from build123d import *

# Parameters (mm, degrees)
SKETCH1_R           = 1.575
SKETCH1_W           = 3
SKETCH1_H           = 8
BOSS_EXTRUDE1_DEPTH = 3
SKETCH1_3_W         = 3
SKETCH1_3_H         = 8
SKETCH1_3_W_2       = 1.7
BOSS_EXTRUDE2_DEPTH = 15
SKETCH1_4_W         = 11.6
SKETCH1_4_H         = 3
BOSS_EXTRUDE3_DEPTH = 3.8
FILLET1_R           = 3


with BuildPart() as part:
    # Sketch1 → Boss-Extrude1 (new body)
    with BuildSketch(Plane(origin=(0, 0, 0), x_dir=(1, 0, 0), z_dir=(0, 1, 0))):
        Polygon((-13.5, -21.27), (-19.3, -28.36), (13.5, -28.36), (13.5, -20.375), (11.8, -20.375), (11.8, -12.375), (13.5, -12.375), (13.5, 12.375), (11.8, 12.375), (11.8, 20.375), (13.5, 20.375), (13.5, 28.36), (-19.3, 28.36), (-13.5, 21.27), align=None)
        with Locations(Location((-8.738402562, -18, 0), (0, 0, 270))):
            Circle(SKETCH1_R, mode=Mode.SUBTRACT)
        with Locations(Location((3.261597438, -18, 0), (0, 0, 270))):
            Circle(SKETCH1_R, mode=Mode.SUBTRACT)
        with Locations((7, -16.375)):
            Rectangle(SKETCH1_W, SKETCH1_H, mode=Mode.SUBTRACT)
        with Locations(Location((-8.738402562, 18, 0), (0, 0, 270))):
            Circle(SKETCH1_R, mode=Mode.SUBTRACT)
        with Locations(Location((3.261597438, 18, 0), (0, 0, 270))):
            Circle(SKETCH1_R, mode=Mode.SUBTRACT)
        with Locations((7, 16.375)):
            Rectangle(SKETCH1_W, SKETCH1_H, mode=Mode.SUBTRACT)
    extrude(amount=BOSS_EXTRUDE1_DEPTH)

    # Sketch1_3 → Boss-Extrude2 (add)
    with BuildSketch(Plane(origin=(0, 0, 0), x_dir=(1, 0, 0), z_dir=(0, 1, 0))):
        with Locations((7, 16.375)):
            Rectangle(SKETCH1_3_W, SKETCH1_3_H)
        with Locations((7, -16.375)):
            Rectangle(SKETCH1_3_W, SKETCH1_3_H)
        with Locations((12.65, -16.375)):
            Rectangle(SKETCH1_3_W_2, SKETCH1_3_H)
        with Locations((12.65, 16.375)):
            Rectangle(SKETCH1_3_W_2, SKETCH1_3_H)
    extrude(amount=BOSS_EXTRUDE2_DEPTH)

    # Sketch1_4 → Boss-Extrude3 (add)
    with BuildSketch(Plane(origin=(0, 0, 0), x_dir=(1, 0, 0), z_dir=(0, 1, 0))):
        with Locations((-13.5, -29.86)):
            Rectangle(SKETCH1_4_W, SKETCH1_4_H)
        with Locations((-13.5, 29.86)):
            Rectangle(SKETCH1_4_W, SKETCH1_4_H)
    extrude(amount=BOSS_EXTRUDE3_DEPTH)

    # Fillet1
    fillet1_edges = [part.edges().sort_by_distance(p)[0] for p in [
        (13.5, 1.5, 28.36),
        (13.5, 1.5, -28.36),
    ]]
    fillet(fillet1_edges, radius=FILLET1_R)


solid = part.part
Could you check a few things on this model? Use its own coordinates, in mm. A direction names the side the tool comes from. Round coordinates to 2 decimals unless told otherwise and drop trailing zeros. Write each loop counter-clockwise with the first axis right and the second up, starting at its lowest first coordinate (ties: lowest second). Pieces come first, ordered by that corner, then holes. Notation, with made-up numbers: (50, 66.5) -> (63, 66.5) arc R36 ccw to (63, 103.5) -> close; hole circle Ø8 at (-30, 37.5). An arc over 180 degrees is marked (long way). Use a Markdown table: item, result.
1. If we section it at A-A (y = 14.25): List the corners of the cut face in (x, z) for me (3 decimals).
Answer key:
| item | result |
|---|---|
| outline | (5.5, -20.375) -> (8.5, -20.375) -> (8.5, -12.375) -> (5.5, -12.375) -> close; (5.5, 12.375) -> (8.5, 12.375) -> (8.5, 20.375) -> (5.5, 20.375) -> close; (11.8, -20.375) -> (13.5, -20.375) -> (13.5, -12.375) -> (11.8, -12.375) -> close; (11.8, 12.375) -> (13.5, 12.375) -> (13.5, 20.375) -> (11.8, 20.375) -> close |
2. Which directions (+Z, -Z, +X, -X, +Y, -Y) give clear straight access to the entire face, cutting with the end or side of a thin tool? Please do faces 5 (the face through (7, 9, -20.375)), 6 (the face through (7, 9, 12.375)), 7 (the face through (13, 9, 20.375)), 8 (the face through (2, 1, -28.36)), 9 (the face through (11.8, 9, 16)).
Answer key:
| item | result |
|---|---|
| face 5 | -Z, +X, -X, +Y |
| face 6 | +X, -X, +Y |
| face 7 | +Z, +X, -X, +Y |
| face 8 | -Z, +X, +Y, -Y |
| face 9 | +Z, -Z, +Y |
3. Please list where these lines run through material, in increasing order: probe 1 along X at (y, z) = (2.3, 18); probe 2 along X at (y, z) = (13, 16.5); probe 3 along X at (y, z) = (1.25, -18.5).
Answer key:
| item | result |
|---|---|
| probe 1 | x = -13.5 to -10.31, -7.16 to 1.69, 4.84 to 13.5 |
| probe 2 | x = 5.5 to 8.5, 11.8 to 13.5 |
| probe 3 | x = -13.5 to -10.23, -7.24 to 1.77, 4.76 to 13.5 |
4. If we section it at B-B (z = -18): List the corners of the cut face in (x, y) for me, then the cut area to 4 significant figures.
Answer key:
| item | result |
|---|---|
| outline | (-13.5, 0) -> (-10.31, 0) -> (-10.31, 3) -> (-13.5, 3) -> close; (-7.16, 0) -> (1.69, 0) -> (1.69, 3) -> (-7.16, 3) -> close; (4.84, 0) -> (13.5, 0) -> (13.5, 15) -> (11.8, 15) -> (11.8, 3) -> (8.5, 3) -> (8.5, 15) -> (5.5, 15) -> (5.5, 3) -> (4.84, 3) -> close |
| area | 118.5 mm^2 |
5. For pin 1 Ø2.5 at (y, z) = (1.5, -2) entering from -X; pin 2 Ø8 at (x, z) = (-13, 6.5) entering from +Y; pin 3 Ø3.5 at (x, y) = (7, 11.5) entering from -Z (3 decimals), each with a flat end and sliding along its axis, tell me the tip position at first contact or that it passes through.
Answer key:
| item | result |
|---|---|
| pin 1 | stops at x = -13.5 |
| pin 2 | stops at y = 3 |
| pin 3 | stops at z = -20.375 |
6. We'd pull the mould along X, two halves only. Please class faces 1 (the face through (3.735, 1.479, -16.498)), 2 (the face through (1, 0, 0)), 3 (the face through (-10.136, 1.479, -17.273)), 4 (the face through (-13.5, 1, 0)): +X half, -X half, draft (parallel to the pull), parting line (faces both ways), or undercut.
Answer key:
| item | result |
|---|---|
| face 1 | undercut |
| face 2 | draft |
| face 3 | undercut |
| face 4 | -X half |
7. If we section it at C-C (x = 2.5): List the corners of the cut face in (y, z) for me.
Answer key:
| item | result |
|---|---|
| outline | (0, -28.36) -> (3, -28.36) -> (3, -19.38) -> (0, -19.38) -> close; (0, -16.62) -> (3, -16.62) -> (3, 16.62) -> (0, 16.62) -> close; (0, 19.38) -> (3, 19.38) -> (3, 28.36) -> (0, 28.36) -> close |
